from build123d import *

# Parameters (mm, degrees)
F0_W     = 80
F0_H     = 84
F1_DEPTH = 38
F2_T     = -2.5
F3_R     = 5


with BuildPart() as f1:
    # F0 (on Top) → F1 (new body)
    with BuildSketch(Plane.XY):
        with Locations((-40, 42)):
            Rectangle(F0_W, F0_H)
    extrude(amount=F1_DEPTH)

    # F2
    f2_openings = [f1.faces().sort_by_distance(p)[0] for p in [
        (-40, 42, 38),
    ]]
    offset(amount=F2_T, openings=f2_openings)

    # F3
    f3_edges = [f1.edges().sort_by_distance(p)[0] for p in [
        (-77.5, 81.5, 20.25),
        (-2.5, 81.5, 20.25),
        (-2.5, 2.5, 20.25),
        (-77.5, 2.5, 20.25),
    ]]
    fillet(f3_edges, radius=F3_R)


solid = f1.part
Model file for the job. Use its own axes, mm. A direction names the side the tool comes from. Give positions to 0.01 mm unless a question says otherwise; leave off trailing zeros. Loops run counter-clockwise (first coordinate to the right, second up) from the corner with the lowest first, then second, coordinate; pieces in that order, holes last.
1) Saw through at B-B (x = -22.5). Write the cut outline in (y, z), plus the area to 4 significant figures.
2) Flat gauge pin, fed straight in: pin 1 Ø8 at (x, y) = (-60.5, 38) entering from +Z. Where does the tip first touch, or does it go through?
3) Saw through at A-A (z = 22.5). Write the cut outline in (x, y).
4) Tool access for faces 4 (the cylindrical face through (-4, 3.93, 20.5)), 5 (the flat face through (-41, 84, 19)): list every direction of +Z, -Z, +X, -X, +Y, -Y with a clear straight run to the whole face (end or side of a thin tool).
5) Pull direction X, two halves, no side cores. Call faces 1 (the flat face through (-41, 0, 19)), 2 (the cylindrical face through (-3.93, 80, 20)), 3 (the flat face through (-80, 41, 19)): +X half, -X half, draft (parallel to the pull), parting line (faces both ways), or undercut.
6) Wall check: line 1 (X direction, y = 28, z = 4); line 2 (Y direction, x = -29, z = 21); line 3 (Z direction, x = -5, y = 31.5). Give the ranges that are in metal, low to high.
7) Saw through at C-C (y = 49). Write the cut outline in (x, z), plus the area to 4 significant figures.
Answer block:
1. outline: (0, 0) - (84, 0) - (84, 38) - (81.5, 38) - (81.5, 2.5) - (2.5, 2.5) - (2.5, 38) - (0, 38) - close
1. area: 387.5 mm2
2. pin 1: stops at z = 2.5
3. outline: (-80, 0) - (0, 0) - (0, 84) - (-80, 84) - close; hole (-77.5, 7.5) arc R5 ccw to (-72.5, 2.5) - (-7.5, 2.5) arc R5 ccw to (-2.5, 7.5) - (-2.5, 76.5) arc R5 ccw to (-7.5, 81.5) - (-72.5, 81.5) arc R5 ccw to (-77.5, 76.5) - close
4. face 4: +Z
4. face 5: +Z, -Z, +X, -X, +Y
5. face 1: draft
5. face 2: undercut
5. face 3: -X half
6. line 1: x = -80 to -77.5, -2.5 to 0
6. line 2: y = 0 to 2.5, 81.5 to 84
6. line 3: z = 0 to 2.5
7. outline: (-80, 0) - (0, 0) - (0, 38) - (-2.5, 38) - (-2.5, 2.5) - (-77.5, 2.5) - (-77.5, 38) - (-80, 38) - close
7. area: 377.5 mm2
